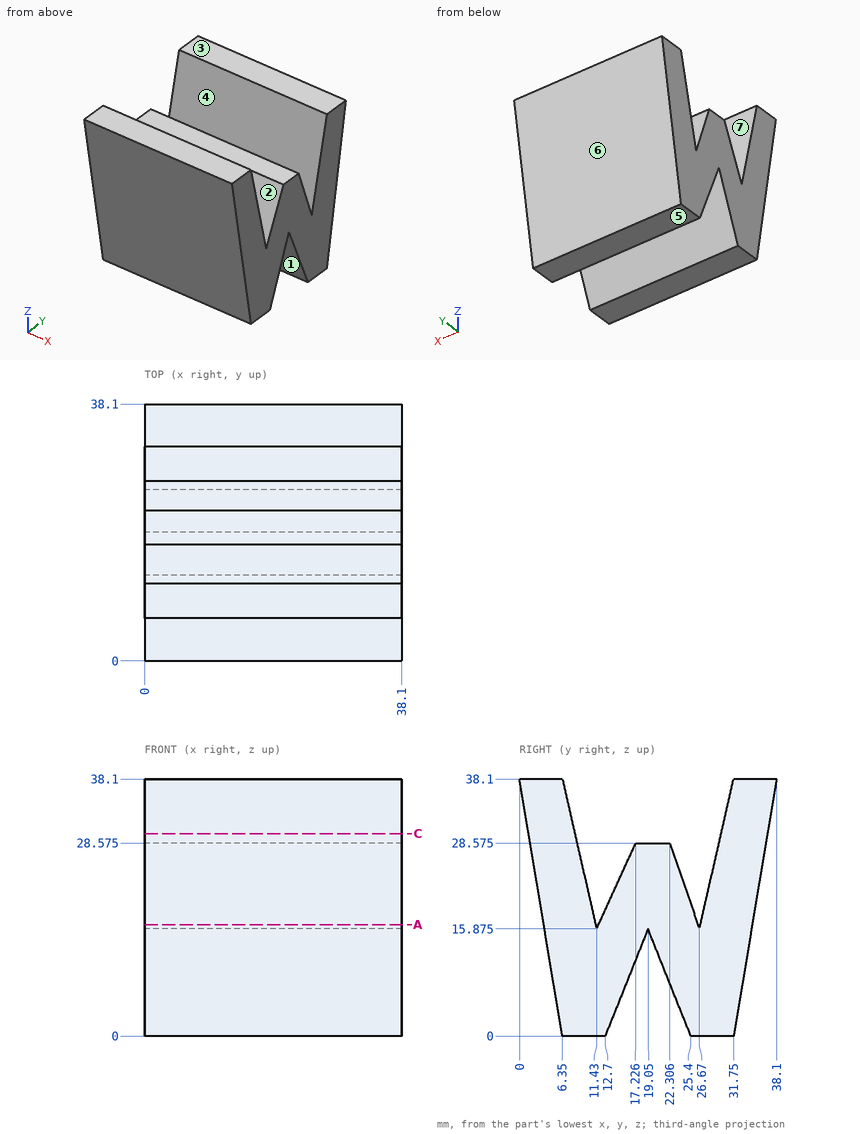
Drawing for the job (mm, zero at the part's lowest x, y, z). A direction names the side the tool comes from. Round coordinates to 2 decimals unless told otherwise and drop trailing zeros. Write each loop counter-clockwise with the first axis right and the second up, starting at its lowest first coordinate (ties: lowest second). Pieces come first, ordered by that corner, then holes. Notation, with made-up numbers: M 78,83.5 L 104,83.5 A19 cw 104,109.5 Z; hole C 88,21.5 d4. An arc over 180 degrees is marked long. Put each result on its own line as item: value.
Item 1: Tool access for the marked faces 1, 2 and 3: list every direction of +Z, -Z, +X, -X, +Y, -Y with a clear straight run to the whole face (end or side of a thin tool).
Responses:
face 1: -Z, +X, -X
face 2: +Z, +X, -X
face 3: +Z, +X, -X, +Y, -Y
Item 2: Cut at C-C (z = 30). List the corners of the cut face in (x, y).
Responses:
outline: M 0,1.35 L 38.1,1.35 L 38.1,8.2 L 0,8.2 Z; M 0,29.9 L 38.1,29.9 L 38.1,36.75 L 0,36.75 Z
Item 3: Flat gauge pins, fed straight in: P1, Ø1, axis at x = 14, z = 28, coming from the -Y side; P2, Ø4, axis at x = 10, y = 20.5, coming from the +Z side (3 decimals); P3, Ø1, axis at x = 20, z = 32, coming from the +Y side. Where does each tip first touch, or does it go through?
Responses:
P1: y = 1.6
P2: z = 28.575
P3: y = 37.17
Item 4: Cut at A-A (z = 16.5). List the corners of the cut face in (x, y) (1 decimal).
Responses:
outline: M 0,3.6 L 38.1,3.6 L 38.1,11.3 L 0,11.3 Z; M 0,11.7 L 38.1,11.7 L 38.1,26.5 L 0,26.5 Z; M 0,26.8 L 38.1,26.8 L 38.1,34.5 L 0,34.5 Z
Item 5: Mould opens along Y. For the marked faces 4, 5, 6 and 7 say: +Y half, -Y half, draft (parallel to the pull), parting line (faces both ways), or undercut.
Responses:
face 4: undercut
face 5: draft
face 6: +Y half
face 7: undercut
Item 6: Probe L1, parallel to Y at x = 5, z = 28; L2, parallel to Y at x = 28, z = 25 (1 decimal); L3, parallel to Y at x = 11.5, z = 4. List the from-to ranges inside material, lowest first. Write a range as from..to.
Responses:
L1: 1.68..8.66, 16.96..22.5, 29.44..36.42
L2: 2.2..9.3, 15.6..23.5, 28.8..35.9
L3: 5.68..14.3, 23.8..32.42
